Can you work these out from the model? Positions are in its coordinate system, mm. Give positions to 0.01 mm unless a question says otherwise; leave off trailing zeros. Loops run counter-clockwise (first coordinate to the right, second up) from the corner with the lowest first, then second, coordinate; pieces in that order, holes last. Notation, with made-up numbers: M 65.5,83.5 L 119.5,83.5 A14 cw 119.5,88.5 Z; hole C -20,64.25 d3. An arc over 180 degrees is marked long. Answer as a JSON object with one key per item and string values.
Autodesk Inventor part; units mm, degrees
ref_plane "YZ Plane" through (0, 0, 0) normal (1, 0, 0) x (0, 1, 0)
ref_plane "XZ Plane" through (0, 0, 0) normal (0, 1, 0) x (-1, 0, 0)
ref_plane "XY Plane" through (0, 0, 0) normal (0, 0, 1) x (1, 0, 0)
sketch "Sketch1" plane through (0, 0, 0) normal (0, 0, 1) x (1, 0, 0)
  line L0 (-235, 100) -> (235, 100)
  line L1 (235, 100) -> (235, -100)
  line L2 (235, -100) -> (-235, -100)
  line L3 (-235, -100) -> (-235, 100)
  line L4 (-235, 100) -> (235, -100) construction
  line L5 (235, 100) -> (-235, -100) construction
  line L6 (-15, 94) -> (15, 94)
  line L7 (15, 94) -> (15, 100)
  line L8 (15, 100) -> (-15, 100)
  line L9 (-15, 100) -> (-15, 94)
  line L10 (-15, 94) -> (15, 100) construction
  line L11 (15, 94) -> (-15, 100) construction
  line L12 (45, 94) -> (75, 94)
  line L13 (75, 94) -> (75, 100)
  line L14 (75, 100) -> (45, 100)
  line L15 (45, 100) -> (45, 94)
  line L16 (45, 94) -> (75, 100) construction
  line L17 (75, 94) -> (45, 100) construction
  line L18 (105, 94) -> (135, 94)
  line L19 (135, 94) -> (135, 100)
  line L20 (135, 100) -> (105, 100)
  line L21 (105, 100) -> (105, 94)
  line L22 (105, 94) -> (135, 100) construction
  line L23 (135, 94) -> (105, 100) construction
  line L24 (165, 94) -> (195, 94)
  line L25 (195, 94) -> (195, 100)
  line L26 (195, 100) -> (165, 100)
  line L27 (165, 100) -> (165, 94)
  line L28 (165, 94) -> (195, 100) construction
  line L29 (195, 94) -> (165, 100) construction
  line L30 (-75, 94) -> (-45, 94)
  line L31 (-45, 94) -> (-45, 100)
  line L32 (-45, 100) -> (-75, 100)
  line L33 (-75, 100) -> (-75, 94)
  line L34 (-75, 94) -> (-45, 100) construction
  line L35 (-45, 94) -> (-75, 100) construction
  line L36 (-15, 94) -> (15, 94)
  line L37 (15, 94) -> (15, 100)
  line L38 (15, 100) -> (-15, 100)
  line L39 (-15, 100) -> (-15, 94)
  line L40 (-15, 94) -> (15, 100) construction
  line L41 (15, 94) -> (-15, 100) construction
  line L42 (45, 94) -> (75, 94)
  line L43 (75, 94) -> (75, 100)
  line L44 (75, 100) -> (45, 100)
  line L45 (45, 100) -> (45, 94)
  line L46 (45, 94) -> (75, 100) construction
  line L47 (75, 94) -> (45, 100) construction
  line L48 (105, 94) -> (135, 94)
  line L49 (135, 94) -> (135, 100)
  line L50 (135, 100) -> (105, 100)
  line L51 (105, 100) -> (105, 94)
  line L52 (105, 94) -> (135, 100) construction
  line L53 (135, 94) -> (105, 100) construction
  line L54 (-135, 94) -> (-105, 94)
  line L55 (-105, 94) -> (-105, 100)
  line L56 (-105, 100) -> (-135, 100)
  line L57 (-135, 100) -> (-135, 94)
  line L58 (-135, 94) -> (-105, 100) construction
  line L59 (-105, 94) -> (-135, 100) construction
  line L60 (-75, 94) -> (-45, 94)
  line L61 (-45, 94) -> (-45, 100)
  line L62 (-45, 100) -> (-75, 100)
  line L63 (-75, 100) -> (-75, 94)
  line L64 (-75, 94) -> (-45, 100) construction
  line L65 (-45, 94) -> (-75, 100) construction
  line L66 (-15, 94) -> (15, 94)
  line L67 (15, 94) -> (15, 100)
  line L68 (15, 100) -> (-15, 100)
  line L69 (-15, 100) -> (-15, 94)
  line L70 (-15, 94) -> (15, 100) construction
  line L71 (15, 94) -> (-15, 100) construction
  line L72 (45, 94) -> (75, 94)
  line L73 (75, 94) -> (75, 100)
  line L74 (75, 100) -> (45, 100)
  line L75 (45, 100) -> (45, 94)
  line L76 (45, 94) -> (75, 100) construction
  line L77 (75, 94) -> (45, 100) construction
  line L78 (-195, 94) -> (-165, 94)
  line L79 (-165, 94) -> (-165, 100)
  line L80 (-165, 100) -> (-195, 100)
  line L81 (-195, 100) -> (-195, 94)
  line L82 (-195, 94) -> (-165, 100) construction
  line L83 (-165, 94) -> (-195, 100) construction
  line L84 (-135, 94) -> (-105, 94)
  line L85 (-105, 94) -> (-105, 100)
  line L86 (-105, 100) -> (-135, 100)
  line L87 (-135, 100) -> (-135, 94)
  line L88 (-135, 94) -> (-105, 100) construction
  line L89 (-105, 94) -> (-135, 100) construction
  line L90 (-75, 94) -> (-45, 94)
  line L91 (-45, 94) -> (-45, 100)
  line L92 (-45, 100) -> (-75, 100)
  line L93 (-75, 100) -> (-75, 94)
  line L94 (-75, 94) -> (-45, 100) construction
  line L95 (-45, 94) -> (-75, 100) construction
  line L96 (-15, 94) -> (15, 94)
  line L97 (15, 94) -> (15, 100)
  line L98 (15, 100) -> (-15, 100)
  line L99 (-15, 100) -> (-15, 94)
  line L100 (-15, 94) -> (15, 100) construction
  line L101 (15, 94) -> (-15, 100) construction
  line L102 (229, -20) -> (235, -20)
  line L103 (235, -20) -> (235, 20)
  line L104 (235, 20) -> (229, 20)
  line L105 (229, 20) -> (229, -20)
  line L106 (229, -20) -> (235, 20) construction
  line L107 (235, -20) -> (229, 20) construction
  line L108 (235, 100) -> (229, 100)
  line L109 (229, 100) -> (229, 60)
  line L110 (229, 60) -> (235, 60)
  line L111 (235, 60) -> (235, 100)
  line L112 (235, -100) -> (229, -100)
  line L113 (229, -100) -> (229, -60)
  line L114 (229, -60) -> (235, -60)
  line L115 (235, -60) -> (235, -100)
  line L116 (0, 100) -> (0, -100) construction
  line L117 (235, 0) -> (-235, 0) construction
  line L118 (-229, -20) -> (-235, -20)
  line L119 (-235, -20) -> (-235, 20)
  line L120 (-235, 20) -> (-229, 20)
  line L121 (-229, 20) -> (-229, -20)
  line L122 (-229, -20) -> (-235, 20) construction
  line L123 (-235, -20) -> (-229, 20) construction
  line L124 (-235, 100) -> (-229, 100)
  line L125 (-229, 100) -> (-229, 60)
  line L126 (-229, 60) -> (-235, 60)
  line L127 (-235, 60) -> (-235, 100)
  line L128 (-235, -100) -> (-229, -100)
  line L129 (-229, -100) -> (-229, -60)
  line L130 (-229, -60) -> (-235, -60)
  line L131 (-235, -60) -> (-235, -100)
  line L132 (-15, -94) -> (15, -94)
  line L133 (15, -94) -> (15, -100)
  line L134 (15, -100) -> (-15, -100)
  line L135 (-15, -100) -> (-15, -94)
  line L136 (-15, -94) -> (15, -100) construction
  line L137 (15, -94) -> (-15, -100) construction
  line L138 (45, -100) -> (45, -94)
  line L139 (45, -94) -> (75, -94)
  line L140 (75, -100) -> (45, -100)
  line L141 (45, -94) -> (75, -100) construction
  line L142 (75, -94) -> (45, -100) construction
  line L143 (75, -94) -> (75, -100)
  line L144 (105, -100) -> (105, -94)
  line L145 (105, -94) -> (135, -94)
  line L146 (135, -100) -> (105, -100)
  line L147 (105, -94) -> (135, -100) construction
  line L148 (135, -94) -> (105, -100) construction
  line L149 (135, -94) -> (135, -100)
  line L150 (165, -100) -> (165, -94)
  line L151 (165, -94) -> (195, -94)
  line L152 (195, -100) -> (165, -100)
  line L153 (165, -94) -> (195, -100) construction
  line L154 (195, -94) -> (165, -100) construction
  line L155 (195, -94) -> (195, -100)
  line L156 (-75, -100) -> (-75, -94)
  line L157 (-75, -94) -> (-45, -94)
  line L158 (-45, -100) -> (-75, -100)
  line L159 (-75, -94) -> (-45, -100) construction
  line L160 (-45, -94) -> (-75, -100) construction
  line L161 (-45, -94) -> (-45, -100)
  line L162 (-15, -100) -> (-15, -94)
  line L163 (-15, -94) -> (15, -94)
  line L164 (15, -100) -> (-15, -100)
  line L165 (-15, -94) -> (15, -100) construction
  line L166 (15, -94) -> (-15, -100) construction
  line L167 (15, -94) -> (15, -100)
  line L168 (45, -100) -> (45, -94)
  line L169 (45, -94) -> (75, -94)
  line L170 (75, -100) -> (45, -100)
  line L171 (45, -94) -> (75, -100) construction
  line L172 (75, -94) -> (45, -100) construction
  line L173 (75, -94) -> (75, -100)
  line L174 (105, -100) -> (105, -94)
  line L175 (105, -94) -> (135, -94)
  line L176 (135, -100) -> (105, -100)
  line L177 (105, -94) -> (135, -100) construction
  line L178 (135, -94) -> (105, -100) construction
  line L179 (135, -94) -> (135, -100)
  line L180 (-135, -100) -> (-135, -94)
  line L181 (-135, -94) -> (-105, -94)
  line L182 (-105, -100) -> (-135, -100)
  line L183 (-135, -94) -> (-105, -100) construction
  line L184 (-105, -94) -> (-135, -100) construction
  line L185 (-105, -94) -> (-105, -100)
  line L186 (-75, -100) -> (-75, -94)
  line L187 (-75, -94) -> (-45, -94)
  line L188 (-45, -100) -> (-75, -100)
  line L189 (-75, -94) -> (-45, -100) construction
  line L190 (-45, -94) -> (-75, -100) construction
  line L191 (-45, -94) -> (-45, -100)
  line L192 (-15, -100) -> (-15, -94)
  line L193 (-15, -94) -> (15, -94)
  line L194 (15, -100) -> (-15, -100)
  line L195 (-15, -94) -> (15, -100) construction
  line L196 (15, -94) -> (-15, -100) construction
  line L197 (15, -94) -> (15, -100)
  line L198 (45, -100) -> (45, -94)
  line L199 (45, -94) -> (75, -94)
  line L200 (75, -100) -> (45, -100)
  line L201 (45, -94) -> (75, -100) construction
  line L202 (75, -94) -> (45, -100) construction
  line L203 (75, -94) -> (75, -100)
  line L204 (-195, -100) -> (-195, -94)
  line L205 (-195, -94) -> (-165, -94)
  line L206 (-165, -100) -> (-195, -100)
  line L207 (-195, -94) -> (-165, -100) construction
  line L208 (-165, -94) -> (-195, -100) construction
  line L209 (-165, -94) -> (-165, -100)
  line L210 (-135, -100) -> (-135, -94)
  line L211 (-135, -94) -> (-105, -94)
  line L212 (-105, -100) -> (-135, -100)
  line L213 (-135, -94) -> (-105, -100) construction
  line L214 (-105, -94) -> (-135, -100) construction
  line L215 (-105, -94) -> (-105, -100)
  line L216 (-75, -100) -> (-75, -94)
  line L217 (-75, -94) -> (-45, -94)
  line L218 (-45, -100) -> (-75, -100)
  line L219 (-75, -94) -> (-45, -100) construction
  line L220 (-45, -94) -> (-75, -100) construction
  line L221 (-45, -94) -> (-45, -100)
  line L222 (-15, -100) -> (-15, -94)
  line L223 (-15, -94) -> (15, -94)
  line L224 (15, -100) -> (-15, -100)
  line L225 (-15, -94) -> (15, -100) construction
  line L226 (15, -94) -> (-15, -100) construction
  line L227 (15, -94) -> (15, -100)
  point P0 (0, 0)
  point P1 (0, 97)
  point P2 (0, 97)
  point P3 (0, 0)
  point P4 (60, 97)
  point P5 (60, 97)
  point P6 (120, 97)
  point P7 (120, 97)
  point P8 (180, 97)
  point P9 (180, 97)
  point P10 (-60, 97)
  point P11 (-60, 97)
  point P12 (0, 97)
  point P13 (0, 97)
  point P14 (60, 97)
  point P15 (60, 97)
  point P16 (120, 97)
  point P17 (120, 97)
  point P18 (-120, 97)
  point P19 (-120, 97)
  point P20 (-60, 97)
  point P21 (-60, 97)
  point P22 (0, 97)
  point P23 (0, 97)
  point P24 (60, 97)
  point P25 (60, 97)
  point P26 (-180, 97)
  point P27 (-180, 97)
  point P28 (-120, 97)
  point P29 (-120, 97)
  point P30 (-60, 97)
  point P31 (-60, 97)
  point P32 (0, 97)
  point P33 (0, 97)
  point P34 (232, 0)
  point P35 (232, 0)
  point P36 (0, 0)
  point P37 (-232, 0)
  point P38 (-232, 0)
  point P39 (0, -97)
  point P40 (60, -100)
  point P41 (60, -97)
  point P42 (120, -100)
  point P43 (120, -97)
  point P44 (180, -100)
  point P45 (180, -97)
  point P46 (-60, -100)
  point P47 (-60, -97)
  point P48 (0, -97)
  point P49 (60, -100)
  point P50 (60, -97)
  point P51 (120, -100)
  point P52 (120, -97)
  point P53 (-120, -100)
  point P54 (-120, -97)
  point P55 (-60, -100)
  point P56 (-60, -97)
  point P57 (0, -97)
  point P58 (60, -100)
  point P59 (60, -97)
  point P60 (-180, -100)
  point P61 (-180, -97)
  point P62 (-120, -100)
  point P63 (-120, -97)
  point P64 (-60, -100)
  point P65 (-60, -97)
  point P66 (0, -97)
  point P67 (0, 85)
  point P68 (0, 100)
  dimension "d0" = 470
  dimension "d1" = 200
  dimension "d2" = 6
  dimension "d3" = 30
  dimension "d6" = 60
  dimension "d9" = 60
  dimension "d12" = 6
  dimension "d13" = 40
  dimension "d14" = 6
  dimension "d15" = 40
  dimension "d16" = 6
  dimension "d17" = 40
  dimension "d20" = 60
  dimension "d23" = 60
extrude "Plate1" add sketch "Sketch1" along normal blind 6 contours L0 L81 L78 L79 L57 L54 L55 L33 L30 L31 L9 L6 L7 L15 L12 L13 L21 L18 L19 L27 L24 L25 L109 L110 L1 L104 L105 L102 L114 L113 L2 L155 L151 L150 L149 L145 L144 L143 L139 L138 L133 L132 L135 L161 L157 L156 L185 L181 L180 L209 L205 L204 L129 L130 L3 L118 L121 L120 L126 L125
equation "\"d12\" = d2"
equation "\"d15\" = d13"
equation "\"d33\" = Thickness"
equation "\"BendRadius\" = Thickness"
equation "\"BendReliefWidth\" = Thickness"
equation "\"BendReliefDepth\" = 0.5 * Thickness"
equation "\"CornerReliefSize\" = 4 * Thickness"
equation "\"MinimumRemnant\" = 2 * Thickness"
equation "\"TransitionRadius\" = BendRadius"
equation "\"JacobiRadiusSize\" = BendRadius"
equation "\"GapSize\" = Thickness"
properties part number "bovenplaat elektrobox v2" material "Wood (Birch)"
1) Suppose I cut it at B-B, the plane x = -10. Write out the boundary of the cut face in (y, z), and give its area (3 significant figures).
Answer list:
{"outline": "M -94,0 L 94,0 L 94,6 L -94,6 Z", "area": "1,130 mm^2"}
2) Will these pins go through, and if not, where does the flat tip stop? pin 1 Ø1.8 at (x, z) = (233, 3) entering from -Y; pin 2 Ø1.8 at (y, z) = (-98, 4.5) entering from +X; pin 3 Ø1 at (x, y) = (-108, -3.5) entering from -Z; pin 4 Ø3 at (x, z) = (-6, 3) entering from +Y.
Answer list:
{"pin 1": "y = -60", "pin 2": "x = 229", "pin 3": "z = 0", "pin 4": "y = 94"}
3) Suppose I cut it at A-A, the plane y = -74.5. Write out the boundary of the cut face in (x, z).
Answer list:
{"outline": "M -229,0 L 229,0 L 229,6 L -229,6 Z"}
4) Please list where these lines run through material, in increasing order: line 1 along Y through (x, z) = (-175, 4.55); line 2 along X through (y, z) = (9.5, 3). Write a range as from..to.
Answer list:
{"line 1": "-94..94", "line 2": "-229..229"}
